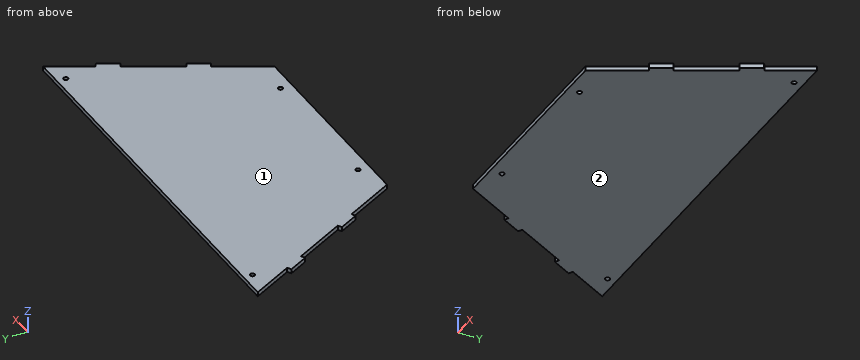
from build123d import *

# Parameters (mm, degrees)
SKETCH_1_R      = 1.6
EXTRUDE_1_DEPTH = 3
SKETCH_2_W      = 3
SKETCH_2_H      = 15
EXTRUDE_2_DEPTH = 3


with BuildPart() as part:
    # 草图1 → 凸台-拉伸1 (new body)
    with BuildSketch(Plane.XY):
        Polygon((-138.666666667, 62), (138.666666667, 62), (72.533333333, -62), (-72.533333333, -62), align=None)
        with Locations((-50, -54)):
            Circle(SKETCH_1_R, mode=Mode.SUBTRACT)
        with Locations((50, -54)):
            Circle(SKETCH_1_R, mode=Mode.SUBTRACT)
        with Locations((-120.466666667, 56)):
            Circle(SKETCH_1_R, mode=Mode.SUBTRACT)
        with Locations((120.466666667, 56)):
            Circle(SKETCH_1_R, mode=Mode.SUBTRACT)
    extrude(amount=EXTRUDE_1_DEPTH)

    # 草图2 → 凸台-拉伸2 (add)
    with BuildSketch(Plane(origin=(-82.214532872, -43.847750865, 0), x_dir=(0, 0, 1), z_dir=(-0.8823529411764701, -0.4705882352941186, 0))):
        with Locations((1.5, 80.460784314)):
            Rectangle(SKETCH_2_W, SKETCH_2_H)
        with Locations((1.5, 25.460784314)):
            Rectangle(SKETCH_2_W, SKETCH_2_H)
    extrude_2 = extrude(amount=EXTRUDE_2_DEPTH)

    # 镜向1: 凸台-拉伸2 across plane
    add(extrude_2.mirror(Plane(origin=(0, 0, 0), x_dir=(0, 0, 1), z_dir=(1, 0, 0))))


solid = part.part
CAD build for the part. Positions are in the model's coordinates, mm. Face numbers are marked on the shaded views. Coordinates: 2 decimals unless noted, no trailing zeros. Write each loop counter-clockwise with the first axis right and the second up, starting at its lowest first coordinate (ties: lowest second). Pieces come first, ordered by that corner, then holes. Notation, with made-up numbers: M 58,88.5 L 103,88.5 A22 cw 103,116.5 Z; hole C 77,-6.75 d3. An arc over 180 degrees is marked long. Return JSON: item names as keys, results as strings.
Item 1: Slice it at B-B, the plane y = -3. Write the cut outline in (x, z), and give its area (3 significant figures).
Findings below:
{"outline": "M -104,0 L 104,0 L 104,3 L -104,3 Z", "area": "624 mm2"}
Item 2: Slice it at A-A, the plane z = 0.9. Write the cut outline in (x, y).
Findings below:
{"outline": "M -138.67,62 L -123.61,33.76 L -126.25,32.35 L -119.2,19.12 L -116.55,20.53 L -97.73,-14.76 L -100.37,-16.18 L -93.31,-29.41 L -90.67,-28 L -72.53,-62 L 72.53,-62 L 90.67,-28 L 93.31,-29.41 L 100.37,-16.18 L 97.73,-14.76 L 116.55,20.53 L 119.2,19.12 L 126.25,32.35 L 123.61,33.76 L 138.67,62 Z; hole C -120.47,56 d3.2; hole C -50,-54 d3.2; hole C 50,-54 d3.2; hole C 120.47,56 d3.2"}
Item 3: Probe line 1 (Y direction, x = -50, z = 2); line 2 (X direction, y = 55.5, z = 1.1); line 3 (Y direction, x = 51, z = 0.3). List the from-to ranges inside material, lowest first. Write a range as from..to.
Findings below:
{"line 1": "y = -62..-55.6, -52.4..62", "line 2": "x = -135.2..-121.99, -118.95..118.95, 121.99..135.2", "line 3": "y = -62..-55.25, -52.75..62"}
Item 4: Two-plate mould, pull along Z, no slides. Class the marked faces 1 and 2: +Z half, -Z half, draft (parallel to the pull), parting line (faces both ways), or undercut.
Findings below:
{"face 1": "+Z half", "face 2": "-Z half"}
Item 5: Drop a flat-ended pin along its axis: pin 1 Ø2.5 at (x, y) = (-120.47, 56) entering from +Z. Give the stop position or say it passes through.
Findings below:
{"pin 1": "passes through"}
Item 6: Slice it at C-C, the plane x = 113. Write the cut outline in (y, z) (3 decimals).
Findings below:
{"outline": "M 13.875,0 L 62,0 L 62,3 L 13.875,3 Z"}
